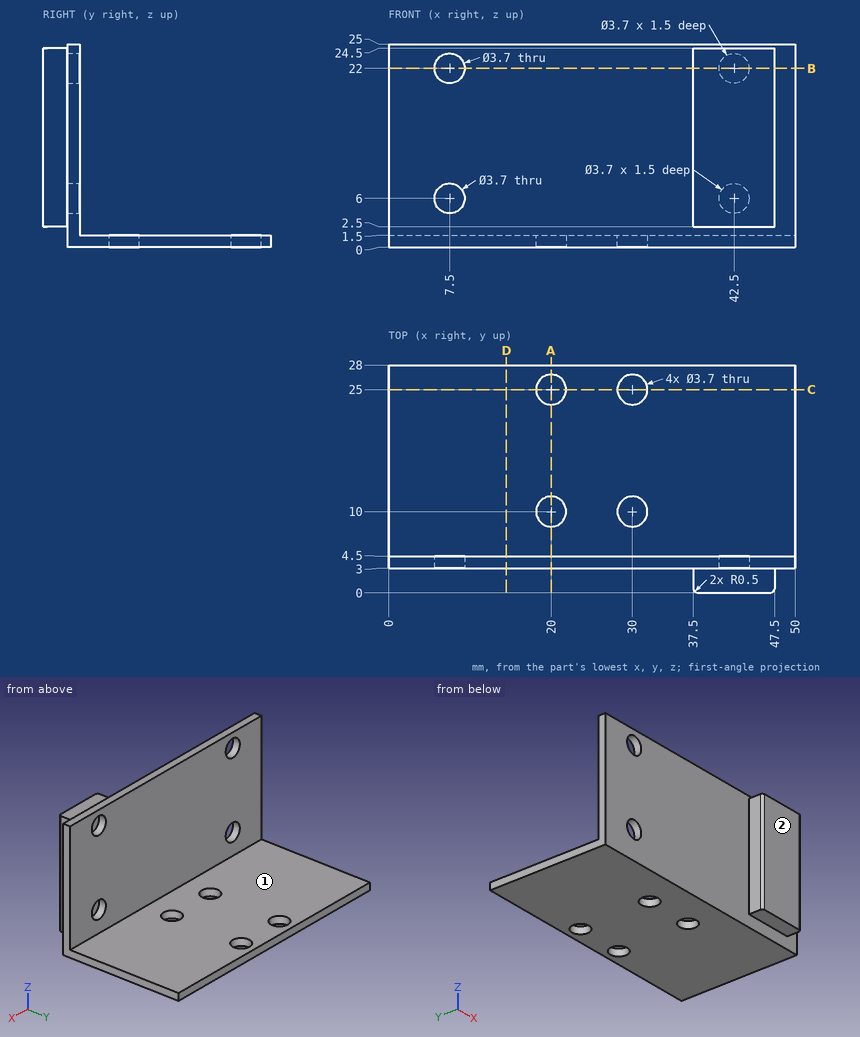
Design review of the part shown in the three views and the two pictorial views. Dimensions are in mm from the part's minimum x, y and z. A direction names the side the tool comes from. Round coordinates to 2 decimals unless told otherwise and drop trailing zeros. Write each loop counter-clockwise with the first axis right and the second up, starting at its lowest first coordinate (ties: lowest second). Pieces come first, ordered by that corner, then holes. Notation, with made-up numbers: (-7.75, -8) - (12.25, -8) arc R37 ccw to (12.25, 30) - close; hole circle Ø4 at (76.25, -38). An arc over 180 degrees is marked (long way). Answer as CSV lines item,"result". Start each with the question number.
(1) Machinability: for the marked faces 1 and 2, which of the approach directions +Z, -Z, +X, -X, +Y, -Y give a long, thin tool a straight path to every point of the face, cutting with its end or side? Answer none if there is none.
(2) Add section D-D, the plane x = 14.5. State the section outline as (y, z) points.
(3) Add section B-B, the plane z = 22. State the section outline as (x, y) points.
(4) Add section A-A, the plane x = 20. State the section outline as (y, z) points.
(5) Add section C-C, the plane y = 25. State the section outline as (x, z) points, plus the area to 3 significant figures.
(6) For line 1 (Z direction, x = 42.5, y = 3.45); line 2 (Y direction, x = 30, z = 0.7); line 3 (X direction, y = 2.5, z = 18.75), list the stretches that pass through material, from the lowest coordinate up.
(7) For pin 1 (0.9 mm diameter, centred on x = 45, y = 1.5, fed in from -Z); pin 2 (6 mm diameter, centred on x = 30, y = 10, fed in from +Z); pin 3 (8 mm diameter, centred on x = 15.5, z = 7, fed in from -Y); pin 4 (3.5 mm diameter, centred on x = 20, y = 10, fed in from +Z), all flat-tipped, find the tip position at first contact; note any pin that passes through.
From the geometry:
1,face 1,"+Z, +X, -X, +Y"
1,face 2,"+Z, -Z, +X, -X, -Y"
2,outline,"(3, 0) - (28, 0) - (28, 1.5) - (4.5, 1.5) - (4.5, 25) - (3, 25) - close"
3,outline,"(0, 3) - (5.65, 3) - (5.65, 4.5) - (0, 4.5) - close; (9.35, 3) - (37.5, 3) - (37.5, 0.5) arc R0.5 ccw to (38, 0) - (47, 0) arc R0.5 ccw to (47.5, 0.5) - (47.5, 3) - (50, 3) - (50, 4.5) - (44.35, 4.5) - (44.35, 3) - (40.65, 3) - (40.65, 4.5) - (9.35, 4.5) - close"
4,outline,"(3, 0) - (8.15, 0) - (8.15, 1.5) - (4.5, 1.5) - (4.5, 25) - (3, 25) - close; (11.85, 0) - (23.15, 0) - (23.15, 1.5) - (11.85, 1.5) - close; (26.85, 0) - (28, 0) - (28, 1.5) - (26.85, 1.5) - close"
5,outline,"(0, 0) - (18.15, 0) - (18.15, 1.5) - (0, 1.5) - close; (21.85, 0) - (28.15, 0) - (28.15, 1.5) - (21.85, 1.5) - close; (31.85, 0) - (50, 0) - (50, 1.5) - (31.85, 1.5) - close"
5,area,"63.9 mm²"
6,line 1,"z = 0 to 4.15, 7.85 to 20.15, 23.85 to 25"
6,line 2,"y = 3 to 8.15, 11.85 to 23.15, 26.85 to 28"
6,line 3,"x = 37.5 to 47.5"
7,pin 1,"stops at z = 2.5"
7,pin 2,"stops at z = 1.5"
7,pin 3,"stops at y = 3"
7,pin 4,"passes through"
